Can you work these out from the model? Positions are in its coordinate system, mm. A direction names the side the tool comes from. Give positions to 0.01 mm unless a question says otherwise; leave off trailing zeros. Order: outer loops, then holes, each group sorted by start corner. A loop starts at its lowest first (then second) coordinate and runs counter-clockwise, first axis right, second up. Notation, with made-up numbers: (49, -12.5) - (84, -12.5) arc R20 cw to (84, -7.5) - close; hole circle Ø1 at (83.5, -13.75). An arc over 180 degrees is marked (long way). Return JSON: item names as keys, results as strings.
```python
from build123d import *

# Parameters (mm, degrees)
SHANK_DIAMETER_R      = 5.55625
SHANK_DEPTH           = 79.375
HEAD_DEPTH            = 6.35
SKETCH1_R             = 1.27
SHANK_HOLE_DEPTH      = 22.828125
SHANK_HOLE_DEPTH_BACK = 5.365625
FILLET1_R             = 0.762
FILLET2_R             = 0.762
CHAMFER1_SIZE         = 0.762
CHAMFER2_SIZE         = 0.127
FILLET4_R             = 0.381


with BuildPart() as part:
    # Shank_Diameter → Shank (new body)
    with BuildSketch(Plane.XY):
        Circle(SHANK_DIAMETER_R)
    extrude(amount=SHANK_DEPTH)

    # Hex 2 → Head (add)
    with BuildSketch(Plane(origin=(0, 0, 0), x_dir=(-1, 0, 0), z_dir=(0, 0, -1))):
        Polygon((-5.040989538, 8.73125), (5.040989538, 8.73125), (10.081979076, 0), (5.040989538, -8.73125), (-5.040989538, -8.73125), (-10.081979076, 0), align=None)
    extrude(amount=HEAD_DEPTH)

    # Sketch1 → Shank_Hole (cut, two sides)
    with BuildSketch(Plane(origin=(-8.305880657, 3.0762927, 0), x_dir=(0, 0, -1), z_dir=(0.866025404, -0.5, 0))) as shank_hole_sk:
        with Locations((-74.6125, 1.4887927)):
            Circle(SKETCH1_R)
    extrude(amount=SHANK_HOLE_DEPTH, mode=Mode.SUBTRACT)
    extrude(shank_hole_sk.sketch, amount=-SHANK_HOLE_DEPTH_BACK, mode=Mode.SUBTRACT)

    # Fillet1
    fillet1_edges = [part.edges().sort_by_distance(p)[0] for p in [
        (5.040989538, 8.73125, -3.175),
        (10.081979076, 0, -3.175),
        (5.040989538, -8.73125, -3.175),
        (-5.040989538, -8.73125, -3.175),
        (-10.081979076, 0, -3.175),
        (-5.040989538, 8.73125, -3.175),
    ]]
    fillet(fillet1_edges, radius=FILLET1_R)

    # Fillet2
    fillet2_edges = [part.edges().sort_by_distance(p)[0] for p in [
        (0, 8.73125, -6.35),
        (-7.561484307, 4.365625, -6.35),
        (7.561484307, 4.365625, -6.35),
        (7.561484307, -4.365625, -6.35),
        (0, -8.73125, -6.35),
        (-7.561484307, -4.365625, -6.35),
    ]]
    fillet(fillet2_edges, radius=FILLET2_R)

    # Chamfer1
    chamfer1_edges = [part.edges().sort_by_distance(p)[0] for p in [
        (-5.55625, 0, 79.375),
    ]]
    chamfer(chamfer1_edges, length=CHAMFER1_SIZE)

    # Chamfer2
    chamfer2_edges = [part.edges().sort_by_distance(p)[0] for p in [
        (0, 8.73125, 0),
        (7.561484307, 4.365625, 0),
        (-7.561484307, 4.365625, 0),
        (-7.561484307, -4.365625, 0),
        (0, -8.73125, 0),
        (7.561484307, -4.365625, 0),
        (-4.982048633, -8.629161358, 0),
        (4.982048633, -8.629161358, 0),
        (-9.964097265, 0, 0),
        (9.964097265, 0, 0),
        (4.982048633, 8.629161358, 0),
        (-4.982048633, 8.629161358, 0),
    ]]
    chamfer(chamfer2_edges, length=CHAMFER2_SIZE)

    # Fillet4
    fillet4_edges = [part.edges().sort_by_distance(p)[0] for p in [
        (-5.55625, 0, 0),
    ]]
    fillet(fillet4_edges, radius=FILLET4_R)


solid = part.part
```
1. On a 3-axis mill with a long thin cutter (end or side, diameter ignored), from which of +Z, -Z, +X, -X, +Y, -Y can I reach the whole of each face in a straight line? I mean faces 5 (the face through (0, 8.731, -3)), 6 (the face through (-4.095, 3.755, 38.949)). Say none if no direction works.
Checks:
{"face 5": "+Z, -Z, +X, -X, +Y", "face 6": "+Z"}
2. For pin 1 Ø10 at (y, z) = (1, 53.5) entering from -X; pin 2 Ø2 at (y, z) = (6, 54) entering from -X; pin 3 Ø1 at (x, z) = (4, 35.5) entering from +Y, each with a flat end and sliding along its axis, tell me the tip position at first contact or that it passes through.
Checks:
{"pin 1": "x = -5.56", "pin 2": "x = -2.42", "pin 3": "y = 4.32"}
3. Suppose I cut it at A-A (z = 23). List the corners of the cut face in (x, y) for me.
Checks:
{"outline": "circle Ø11.11 at (0, 0)"}
4. Thinking about a two-plate mould opening in X: for faces 1 (the face through (0.36, 0.78, 75.55)), 2 (the face through (7.41, -4.2, -6.12)), 3 (the face through (-7.53, 4.42, -2.82)), 4 (the face through (0, 0, -6.35)), which applies, +X half, -X half, draft (parallel to the pull), parting line (faces both ways), or undercut?
Checks:
{"face 1": "undercut", "face 2": "+X half", "face 3": "-X half", "face 4": "draft"}
5. If I drill on L1, parallel to Z at x = -2.75, y = 7.5; L2, parallel to Y at x = 0, z = 31; L3, parallel to X at y = 1.25, z = 37.5, over which ranges is the centre line in solid material (lowest first)? Write a range as [from, to].
Checks:
{"L1": "[-6.35, 0]", "L2": "[-5.56, 5.56]", "L3": "[-5.41, 5.41]"}
